Work out the finished part from the listing and answer in its coordinate system (mm). Round coordinates to 2 decimals unless told otherwise and drop trailing zeros. Order: outer loops, then holes, each group sorted by start corner. A loop starts at its lowest first (then second) coordinate and runs counter-clockwise, first axis right, second up. Notation, with made-up numbers: (-20, -4) - (22, -4) arc R29 ccw to (22, 17) - close; hole circle Ø11 at (-4.5, -6.75). An arc over 180 degrees is marked (long way). Put each result on its own line as item: value.
Autodesk Inventor part; units mm, degrees
ref_plane "YZ Plane" through (0, 0, 0) normal (1, 0, 0) x (0, 1, 0)
ref_plane "XZ Plane" through (0, 0, 0) normal (0, 1, 0) x (-1, 0, 0)
ref_plane "XY Plane" through (0, 0, 0) normal (0, 0, 1) x (1, 0, 0)
sketch "Sketch2" plane through (0, 4, 0) normal (0, 1, 0) x (1, 0, 0)
  circle A0 centre (0, 0) radius 40 construction
  line L0 (15.1987, 37) -> (-15.1987, 37)
  line L1 (-15.1987, 37) -> (-15.1987, 57.3146)
  line L2 (0.2732, 67) -> (10.6706, 67)
  line L3 (15.1987, 57.3127) -> (15.1987, 37)
  line L4 (15.1987, -37) -> (-15.1987, -37)
  line L5 (-15.1987, -37) -> (-15.1987, -57.3146)
  line L6 (0.2732, -67) -> (10.6706, -67)
  line L7 (15.1987, -57.3127) -> (15.1987, -37)
  line L8 (-15.1987, 57.3146) -> (-15.1987, 67)
  line L9 (-15.1987, 67) -> (0.2732, 67)
  line L10 (10.6706, 67) -> (15.1987, 67)
  line L11 (15.1987, 67) -> (15.1987, 57.3127)
  line L12 (0.2732, -67) -> (-15.1987, -67)
  line L13 (-15.1987, -57.3146) -> (-15.1987, -67)
  line L14 (10.6706, -67) -> (15.1987, -67)
  line L15 (15.1987, -67) -> (15.1987, -57.3127)
  circle A1 centre (0, 0) radius 70.9599 construction
  line L16 (-124.5994, 10) -> (53.6394, 112.9062)
  line L17 (70.9599, 102.9062) -> (70.9599, -102.9062)
  point P0 (0, 0)
  dimension "d9" = 80
  dimension "d10" = 74
  dimension "d11" = 30
sketch "Sketch4" plane through (-13.1987, 4, 37) normal (0, 0, 1) x (1, 0, 0)
  circle A0 centre (13.1987, 6) radius 2.75
  circle A1 centre (13.1987, 18) radius 2.75
  line L0 (66.8381, -2) -> (-111.4007, -2)
  line L1 (0, 0) -> (0, 18)
  line L2 (26.3974, 18) -> (26.3974, 0)
  point P0 (13.1987, -4)
  dimension "d35" = 5.5
  dimension "d36" = 12
  dimension "d37" = 8
  dimension "d39" = 26.3974
  dimension "d40" = 13.1987
sketch "Sketch1" plane through (0, 0, 0) normal (0, 1, 0) x (-1, 0, 0)
  line L0 (124.5994, -10) -> (-53.6394, -112.9062)
  line L1 (-70.9599, -102.9062) -> (-70.9599, 102.9062)
  line L2 (-53.6394, 112.9062) -> (124.5994, 10)
  circle A0 centre (0, 0) radius 70.9599 construction
  line L3 (124.5994, 10) -> (124.5994, -10)
  line L4 (-53.6394, -112.9062) -> (-70.9599, -102.9062)
  line L5 (-70.9599, 102.9062) -> (-53.6394, 112.9062)
  circle A1 centre (0, 0) radius 125 construction
  point P0 (141.9199, 0)
  point P1 (-70.9599, -122.9062)
  point P2 (-70.9599, 122.9062)
  dimension "d7" = 250
  dimension "d1" = 20
  dimension "d2" = 20
  dimension "d3" = 20
  dimension "d4" = 20
  dimension "d5" = 20
  dimension "d6" = 20
extrude "Plate1" add sketch "Sketch1" along normal blind 4
sketch "Sketch5" plane through (0, 4, 0) normal (0, 1, 0) x (1, 0, 0)
  circle A0 centre (0, 0) radius 25 construction
  point P0 (-25, 0)
  point P1 (0, 25)
  point P2 (25, 0)
  point P3 (0, -25)
  dimension "d43" = 50
hole "Hole1" at (-25, 4, 0) at (0, 4, -25) at (25, 4, 0) at (0, 4, 25) direction (0, -1, 0) diameter 5.5 end through all
chamfer "Chamfer1" distance 3 angle 45 4 edges at (0, 0, -27.75) (25, 0, -2.75) (-25, 0, -2.75) (0, 0, 22.25)
sketch "Sketch6" plane through (0, 4, 0) normal (0, 1, 0) x (1, 0, 0)
  circle A0 centre (0, 0) radius 114.5994 construction
  line L0 (-124.5994, -10) -> (-124.5994, 10)
  point P0 (-114.5994, 0)
  point P1 (57.2997, -99.246)
  point P2 (57.2997, 99.246)
  dimension "d54" = 10
  dimension "d57" = 360
hole "Hole2" at (57.2997, 4, -99.246) at (57.2997, 4, 99.246) at (-114.5994, 4, 0) direction (0, -1, 0) diameter 6.647 end through all
sketch "Sketch3" plane through (15.1987, 0, 35) normal (0, 0, 1) x (1, 0, 0)
  line L0 (-28.3974, 0) -> (-2, 0)
  line L1 (-2, 0) -> (-2, 30)
  line L2 (-2, 30) -> (-28.3974, 30)
  line L3 (-28.3974, 30) -> (-28.3974, 0)
equation "\"d49\" = Thickness"
equation "\"d40\" = 0.5 * d39"
equation "\"d8\" = Thickness"
equation "\"BendRadius\" = Thickness"
equation "\"BendReliefWidth\" = Thickness"
equation "\"BendReliefDepth\" = 0.5 * Thickness"
equation "\"CornerReliefSize\" = 4 * Thickness"
equation "\"MinimumRemnant\" = 2 * Thickness"
equation "\"TransitionRadius\" = BendRadius"
equation "\"JacobiRadiusSize\" = BendRadius"
equation "\"GapSize\" = Thickness"
properties part number "BasePlate" material "Stainless Steel"
1) Straight lines are drawn through the part: L1, parallel to X at y = 1.65, z = 0; L2, parallel to Z at x = 25, y = 3.6; L3, parallel to Z at x = 0, y = 3.5. For each, find the intervals that lie inside material, in ascending order. Write a range as from..to.
Findings below:
L1: x = -124.6..-117.92, -111.28..-29.1, -20.9..20.9, 29.1..70.96
L2: z = -96.37..-2.75, 2.75..96.37
L3: z = -81.94..-27.75, -22.25..22.25, 27.75..81.94
2) A cutting plane is placed at C-C on z = 25. Write down the section's boundary in (x, y).
Findings below:
outline: (-98.62, 0) - (-5.75, 0) - (-2.75, 3) - (-2.75, 4) - (-98.62, 4) - close; (2.75, 3) - (5.75, 0) - (70.96, 0) - (70.96, 4) - (2.75, 4) - close
3) A cutting plane is placed at D-D on y = 1.1. Write down the section's boundary in (x, z).
Findings below:
outline: (-124.6, -10) - (53.64, -112.91) - (70.96, -102.91) - (70.96, 102.91) - (53.64, 112.91) - (-124.6, 10) - close; hole circle Ø6.65 at (-114.6, 0); hole circle Ø9.3 at (-25, 0); hole circle Ø9.3 at (0, -25); hole circle Ø9.3 at (0, 25); hole circle Ø9.3 at (25, 0); hole circle Ø6.65 at (57.3, -99.25); hole circle Ø6.65 at (57.3, 99.25)
4) A cutting plane is placed at A-A on x = 0. Write down the section's boundary in (y, z), then the cut area to 4 significant figures.
Findings below:
outline: (0, -81.94) - (4, -81.94) - (4, -27.75) - (3, -27.75) - (0, -30.75) - close; (0, -19.25) - (3, -22.25) - (4, -22.25) - (4, 22.25) - (3, 22.25) - (0, 19.25) - close; (0, 30.75) - (3, 27.75) - (4, 27.75) - (4, 81.94) - (0, 81.94) - close
area: 593.5 mm2
5) A cutting plane is placed at B-B on x = -25. Write down the section's boundary in (y, z).
Findings below:
outline: (0, -67.5) - (4, -67.5) - (4, -2.75) - (3, -2.75) - (0, -5.75) - close; (0, 5.75) - (3, 2.75) - (4, 2.75) - (4, 67.5) - (0, 67.5) - close
6) For a pull along Z with two mould halves and no side action, classify faces 1 (the cylindrical face through (22.273, 3.493, -0.358)), 2 (the cylindrical face through (-0.121, 3.493, 22.253)), 3 (the flat face through (-34.232, 1.972, 62.173)), 4 (the flat face through (62.178, 1.972, -107.976)) as pulls with the +Z half, pulls with the -Z half, needs draft (parallel to the pull), parting line crosses it, or undercut.
Findings below:
face 1: undercut
face 2: undercut
face 3: pulls with the +Z half
face 4: pulls with the -Z half
7) Given pin 1 Ø10.5 at (x, z) = (-114.6, 0) entering from -Y; pin 2 Ø1 at (y, z) = (2, -34) entering from -X; pin 3 Ø2 at (y, z) = (2, 74.5) entering from -X; pin 4 Ø6.5 at (x, z) = (25, 0) entering from -Y, each flat-ended and moving along its own axis, determine where each tip first touches the part or whether it passes through.
Findings below:
pin 1: stops at y = 0
pin 2: stops at x = -83.9
pin 3: stops at x = -14.61
pin 4: stops at y = 2.5
